from build123d import *

# Parameters (mm, degrees)
SKETCH1_W            = 110
SKETCH1_H            = 75
BOSS_EXTRUDE1_DEPTH  = 5
SKETCH2_W            = 50.000000309
SKETCH2_H            = 75
BOSS_EXTRUDE2_DEPTH  = 7
SKETCH3_W            = 50.000000309
SKETCH3_H            = 75
BOSS_EXTRUDE3_DEPTH  = 7
SKETCH4_R            = 13.5
CUT_EXTRUDE1_DEPTH   = 133.647088287
SKETCH5_R            = 1.65
CUT_EXTRUDE2_DEPTH   = 7
SKETCH8_R            = 4.025
CUT_EXTRUDE5_DEPTH   = 139.860541663
SKETCH9_W            = 17
SKETCH9_H            = 75
CUT_EXTRUDE6_DEPTH   = 133.647088287
SKETCH13_R           = 2.75
CUT_EXTRUDE7_DEPTH   = 10
SKETCH14_R           = 5
CUT_EXTRUDE8_DEPTH   = 10
BOSS_EXTRUDE4_START  = 2
SKETCH15_W           = 124
SKETCH15_H           = 75
SKETCH15_R           = 2.75
BOSS_EXTRUDE4_DEPTH  = 2
CUT_EXTRUDE11_DEPTH  = 2
MIRROR7_COPY_1_DEPTH = 2
SKETCH20_R           = 2.4
CUT_EXTRUDE12_DEPTH  = 133.647088287
SKETCH21_W           = 110
SKETCH21_H           = 5
BOSS_EXTRUDE5_DEPTH  = 3
FILLET2_R            = 1


with BuildPart() as part:
    # Sketch1 → Boss-Extrude1 (new body)
    with BuildSketch(Plane.XY):
        Rectangle(SKETCH1_W, SKETCH1_H)
    extrude(amount=BOSS_EXTRUDE1_DEPTH)

    # Sketch2 → Boss-Extrude2 (add)
    with BuildSketch(Plane.ZY.offset(55)):
        with Locations((25.000000155, 0)):
            Rectangle(SKETCH2_W, SKETCH2_H)
    extrude(amount=BOSS_EXTRUDE2_DEPTH)

    # Sketch3 → Boss-Extrude3 (add)
    with BuildSketch(Plane(origin=(55, 0, 0), x_dir=(0, 0, -1), z_dir=(1, 0, 0))):
        with Locations((-25.000000155, 0)):
            Rectangle(SKETCH3_W, SKETCH3_H)
    extrude(amount=BOSS_EXTRUDE3_DEPTH)

    # Sketch4 → Cut-Extrude1 (cut, through all)
    with BuildSketch(Plane(origin=(-55, 0, 0), x_dir=(0, 0, -1), z_dir=(1, 0, 0))):
        with Locations((-24, 0)):
            Circle(SKETCH4_R)
    extrude(amount=-CUT_EXTRUDE1_DEPTH, mode=Mode.SUBTRACT)

    # Sketch5 → Cut-Extrude2 (cut)
    with BuildSketch(Plane.ZY.offset(62)):
        with Locations((39.5, 15.5)):
            Circle(SKETCH5_R)
        with Locations((39.5, -15.5)):
            Circle(SKETCH5_R)
        with Locations((8.5, -15.5)):
            Circle(SKETCH5_R)
        with Locations((8.5, 15.5)):
            Circle(SKETCH5_R)
    extrude(amount=-CUT_EXTRUDE2_DEPTH, mode=Mode.SUBTRACT)

    # Sketch8 → Cut-Extrude5 (cut, through all)
    with BuildSketch(Plane.ZY.offset(62)):
        with Locations((24, 30)):
            Circle(SKETCH8_R)
    cut_extrude5 = extrude(amount=-CUT_EXTRUDE5_DEPTH, mode=Mode.SUBTRACT)

    # Mirror1: Cut-Extrude5 across plane
    add(cut_extrude5.mirror(Plane.ZX), mode=Mode.SUBTRACT)

    # Sketch9 → Cut-Extrude6 (cut, through all)
    with BuildSketch(Plane.ZY.offset(-55)):
        with Locations((41.500000309, 0)):
            Rectangle(SKETCH9_W, SKETCH9_H)
    extrude(amount=-CUT_EXTRUDE6_DEPTH, mode=Mode.SUBTRACT)

    # Sketch13 → Cut-Extrude7 (cut)
    with BuildSketch(Plane(origin=(0, 0, 0), x_dir=(-1, 0, 0), z_dir=(0, 0, -1))):
        with Locations((44.25, 19.85)):
            Circle(SKETCH13_R)
        with Locations((2.25, 19.85)):
            Circle(SKETCH13_R)
        with Locations((2.25, -19.85)):
            Circle(SKETCH13_R)
        with Locations((44.25, -19.85)):
            Circle(SKETCH13_R)
    extrude(amount=-CUT_EXTRUDE7_DEPTH, mode=Mode.SUBTRACT)

    # Sketch14 → Cut-Extrude8 (cut)
    with BuildSketch(Plane.ZY.offset(-55)):
        with Locations((24, 0)):
            Circle(SKETCH14_R)
    extrude(amount=-CUT_EXTRUDE8_DEPTH, mode=Mode.SUBTRACT)

    # Sketch15 → Boss-Extrude4 (add)
    with BuildSketch(Plane(origin=(0, 0, 0), x_dir=(-1, 0, 0), z_dir=(0, 0, -1)).offset(BOSS_EXTRUDE4_START)):
        Rectangle(SKETCH15_W, SKETCH15_H)
        with Locations((44.25, 19.85)):
            Circle(SKETCH15_R, mode=Mode.SUBTRACT)
        with Locations((2.25, 19.85)):
            Circle(SKETCH15_R, mode=Mode.SUBTRACT)
        with Locations((2.25, -19.85)):
            Circle(SKETCH15_R, mode=Mode.SUBTRACT)
        with Locations((44.25, -19.85)):
            Circle(SKETCH15_R, mode=Mode.SUBTRACT)
    extrude(amount=-BOSS_EXTRUDE4_DEPTH)

    # Sketch16 → Cut-Extrude11 (cut, symmetric)
    with BuildSketch(Plane(origin=(0, -34.025, 0), x_dir=(1, 0, 0), z_dir=(0, 1, 0))):
        Polygon((58.5, -26.309401386), (60.5, -25.154700847), (60.5, -22.845299771), (58.5, -21.690599232), (56.5, -22.845299771), (56.5, -25.154700847), align=None)
    cut_extrude11 = extrude(amount=CUT_EXTRUDE11_DEPTH, both=True, mode=Mode.SUBTRACT)

    # Sketch18 → Dégagement M21 (revolve, cut)
    with BuildSketch(Plane(origin=(58.5, -37.5, 24.000000309), x_dir=(0, 0, -1), z_dir=(1, 0, 0))):
        Polygon((0, 0), (0, 5.721032743), (1.2, 5), (1.2, 0), align=None)
    d_gagement_m21 = revolve(axis=Axis((58.5, -43.85, 24.000000309), (0, 1, 0)), mode=Mode.SUBTRACT)

    # Mirror5: Cut-Extrude11, Dégagement M21 across plane
    add(cut_extrude11.mirror(Plane(origin=(0, 0, 0), x_dir=(0, 0, 1), z_dir=(1, 0, 0))), mode=Mode.SUBTRACT)
    add(d_gagement_m21.mirror(Plane(origin=(0, 0, 0), x_dir=(0, 0, 1), z_dir=(1, 0, 0))), mode=Mode.SUBTRACT)

    # Mirror7: Cut-Extrude11, Dégagement M21 across plane
    add(cut_extrude11.mirror(Plane.ZX), mode=Mode.SUBTRACT)
    add(d_gagement_m21.mirror(Plane.ZX), mode=Mode.SUBTRACT)

    # Mirror7 copy 1 sketch → Mirror7 copy 1 (cut, symmetric)
    with BuildSketch(Plane(origin=(0, 34.025, 0), x_dir=(-1, 0, 0), z_dir=(0, -1, 0))):
        Polygon((58.5, -26.309401386), (60.5, -25.154700847), (60.5, -22.845299771), (58.5, -21.690599232), (56.5, -22.845299771), (56.5, -25.154700847), align=None)
    extrude(amount=MIRROR7_COPY_1_DEPTH, both=True, mode=Mode.SUBTRACT)

    # Mirror7 copy 2 sketch → Mirror7 copy 2 (revolve, cut)
    with BuildSketch(Plane(origin=(-58.5, 37.5, 24.000000309), x_dir=(0, 0, -1), z_dir=(-1, 0, 0))):
        Polygon((0, 0), (0, 5.721032743), (1.2, 5), (1.2, 0), align=None)
    revolve(axis=Axis((-58.5, 43.85, 24.000000309), (0, -1, 0)), mode=Mode.SUBTRACT)

    # Sketch20 → Cut-Extrude12 (cut, through all)
    with BuildSketch(Plane.ZY.offset(-55)):
        with Locations((24, 18.25)):
            Circle(SKETCH20_R)
        with Locations((24, -18.25)):
            Circle(SKETCH20_R)
    extrude(amount=-CUT_EXTRUDE12_DEPTH, mode=Mode.SUBTRACT)

    # Sketch21 → Boss-Extrude5 (add)
    with BuildSketch(Plane.XY.offset(5)):
        with Locations((0, 35)):
            Rectangle(SKETCH21_W, SKETCH21_H)
        with Locations((0, -35)):
            Rectangle(SKETCH21_W, SKETCH21_H)
    extrude(amount=BOSS_EXTRUDE5_DEPTH)

    # Fillet2
    fillet2_edges = [part.edges().sort_by_distance(p)[0] for p in [
        (55, 0, 5),
        (-55, 0, 5),
        (55, 32.5, 6.5),
        (0, 32.5, 5),
        (-55, 32.5, 6.5),
        (55, 35, 8),
        (-55, 35, 8),
        (-55, -32.5, 6.5),
        (0, -32.5, 5),
        (55, -32.5, 6.5),
        (-55, -35, 8),
        (55, -35, 8),
    ]]
    fillet(fillet2_edges, radius=FILLET2_R)


solid = part.part
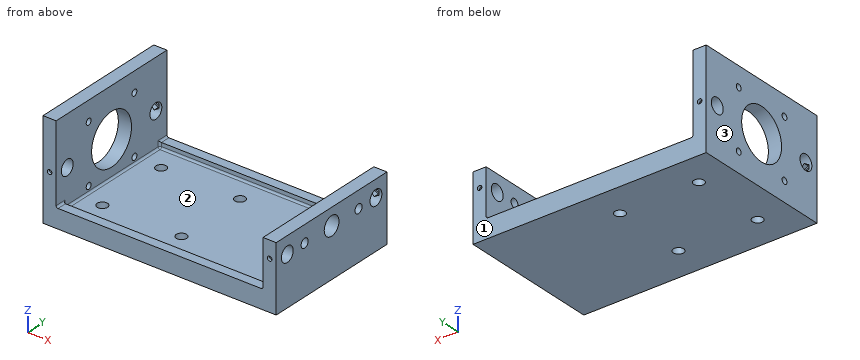
Design review of the part built by this model. Coordinates are the model's own, in mm. Face numbers are marked on the shaded views. Round coordinates to 2 decimals unless told otherwise and drop trailing zeros. Loops run counter-clockwise (first coordinate to the right, second up) from the corner with the lowest first, then second, coordinate; pieces in that order, holes last. Notation, with made-up numbers: (24, 5.25) - (83, 5.25) arc R13 cw to (83, 12.25) - close; hole circle Ø4 at (71.5, 19.5). An arc over 180 degrees is marked (long way). One line per question, with ' | ' between items.
1. For L1, parallel to Y at x = -2.25, z = 0; L2, parallel to X at y = 19.5, z = 7; L3, parallel to Y at x = -59.25, z = 8.5, list the stretches that pass through material, from the lowest coordinate up. Write a range as [from, to].
Results are:
L1: y = [-37.5, -22.6], [-17.1, 17.1], [22.6, 37.5] | L2: x = [-62, -55], [55, 62] | L3: y = [-37.5, -17.15], [-13.85, 13.85], [17.15, 37.5]
2. Draft analysis for pull direction X (two halves, no side actions). For the marked faces 1, 2 and 3, state which applies: released by +X, released by -X, zero draft, split by the parting line, or undercut.
Results are:
face 1: zero draft | face 2: undercut | face 3: released by -X
3. We need section B-B, the plane x = 6.5. State the section outline as (y, z) points.
Results are:
outline: (-37.5, -2) - (37.5, -2) - (37.5, 8) - (32.5, 8) - (32.5, 6) arc R1 cw to (31.5, 5) - (-31.5, 5) arc R1 cw to (-32.5, 6) - (-32.5, 8) - (-37.5, 8) - close
4. We need section A-A, the plane y = -30. State the section outline as (x, z) points (3 decimals).
Results are:
outline: (-62, -2) - (62, -2) - (62, 19.975) - (55, 19.975) - (55, 6) arc R1 cw to (54, 5) - (-54, 5) arc R1 cw to (-55, 6) - (-55, 19.975) - (-62, 19.975) - close; (-62, 28.025) - (-55, 28.025) - (-55, 50) - (-62, 50) - close; (55, 28.025) - (62, 28.025) - (62, 33) - (55, 33) - close
5. Clearance check with flat-ended pins moving along their axes: P1, Ø12, axis at x = -42.5, y = -13, coming from the +Z side; P2, Ø2.5, axis at x = -4.5, y = 36, coming from the +Z side; P3, Ø21.5, axis at y = 1, z = 21.5, coming from the -X side. State where each tip first meets the part, or that it passes through.
Results are:
P1: stops at z = 5 | P2: stops at z = 8 | P3: stops at x = 55
6. We need section C-C, the plane y = 0. State the section outline as (x, z) points, and give its area (3 significant figures).
Results are:
outline: (-62, -2) - (62, -2) - (62, 19) - (55, 19) - (55, 6) arc R1 cw to (54, 5) - (-54, 5) arc R1 cw to (-55, 6) - (-55, 10.5) - (-62, 10.5) - close; (-62, 37.5) - (-55, 37.5) - (-55, 50) - (-62, 50) - close; (55, 29) - (62, 29) - (62, 33) - (55, 33) - close | area: 1,120 mm²
7. We need section D-D, the plane z = 42.5. State the section outline as (x, y) points.
Results are:
outline: (-62, -37.5) - (-55, -37.5) - (-55, 37.5) - (-62, 37.5) - close
